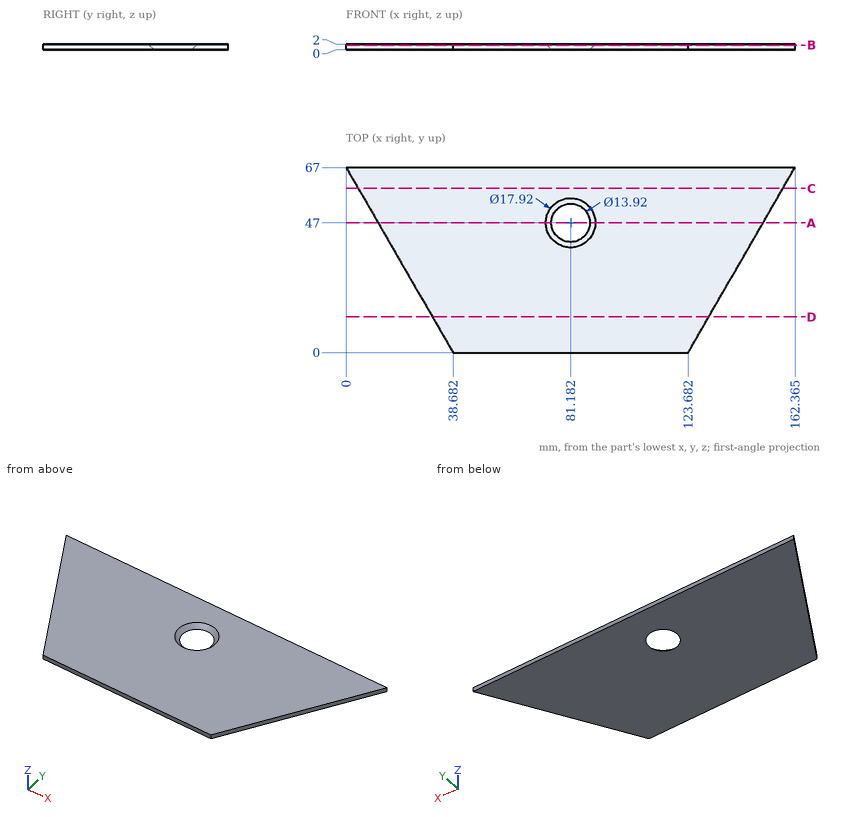
Source: three-view drawing plus pictorial views. Frame: mm from the lowest corner of the part. Coordinates: 2 decimals unless noted, no trailing zeros. Loops run counter-clockwise (first coordinate to the right, second up) from the corner with the lowest first, then second, coordinate; pieces in that order, holes last. Notation, with made-up numbers: (32.25, 33) -> (91.25, 33) arc R15 cw to (91.25, 46) -> close; hole circle Ø3 at (35.25, 72). An arc over 180 degrees is marked (long way). Answer in a Markdown table with one row per item. Add a question column.
Q1. Section D-D on y = 13. Return the cut outline in (x, z).
Q2. Section B-B on z = 1.6. Return the cut outline in (x, y) (1 decimal), and give its area (3 significant figures).
Q3. Contact query for a flat-ended pin moving along its axis: pin 1 Ø1 at (x, z) = (114.5, 1) entering from -Y. Output: stop coordinate, or through.
Q4. Section C-C on y = 59.5. Return the cut outline in (x, z) (1 decimal).
Q5. Section A-A on y = 47. Return the cut outline in (x, z).
Q6. Ray query, line 1 along X through (y, z) = (45, 0.15) (1 decimal); line 2 along X through (y, z) = (57.5, 1.9) (1 decimal); line 3 along Y through (x, z) = (81, 0.55) (1 decimal). Return the intervals inside material, ascending.
Computed values:
| question | item | result |
|---|---|---|
| 1 | outline | (31.18, 0) -> (131.19, 0) -> (131.19, 2) -> (31.18, 2) -> close |
| 2 | outline | (0, 67) -> (38.7, 0) -> (123.7, 0) -> (162.4, 67) -> close; hole circle Ø17.1 at (81.2, 47) |
| 2 | area | 8,060 mm^2 |
| 3 | pin 1 | stops at y = 0 |
| 4 | outline | (4.3, 0) -> (158, 0) -> (158, 2) -> (4.3, 2) -> close |
| 5 | outline | (11.55, 0) -> (74.22, 0) -> (72.22, 2) -> (11.55, 2) -> close; (88.14, 0) -> (150.82, 0) -> (150.82, 2) -> (90.14, 2) -> close |
| 6 | line 1 | x = 12.7 to 74.4, 88 to 149.7 |
| 6 | line 2 | x = 5.5 to 156.9 |
| 6 | line 3 | y = 0 to 39.5, 54.5 to 67 |
